from build123d import *

# Parameters (mm, degrees)
SKETCH1_W            = 12
SKETCH1_H            = 30
BOSS_EXTRUDE1_DEPTH  = 3
BOSS_EXTRUDE2_DEPTH  = 13
M5_CLEARANCE_HOLE1_D = 5.5
M4_CLEARANCE_HOLE1_D = 4.5


with BuildPart() as part:
    # Sketch1 → Boss-Extrude1 (new body)
    with BuildSketch(Plane.XY):
        with Locations((6, 15)):
            Rectangle(SKETCH1_W, SKETCH1_H)
        Polygon((12, 0), (0, 0), (0, -3), (30, -3), (30, 0), align=None)
    extrude(amount=BOSS_EXTRUDE1_DEPTH)

    # Sketch1_3 → Boss-Extrude2 (add)
    with BuildSketch(Plane.XY):
        Polygon((12, 0), (0, 0), (0, -3), (30, -3), (30, 0), align=None)
    extrude(amount=-BOSS_EXTRUDE2_DEPTH)

    # Mirror1: part across plane


with BuildPart() as part_1:
    add(part.part)
    add(part.part.mirror(Plane.XY.offset(-13)))

    # M5 Clearance Hole1 (through all)
    with Locations(Plane(origin=(0, 0, 0), x_dir=(1, 0, 0), z_dir=(0, 1, 0))):
        with Locations((20, 13)):
            Hole(M5_CLEARANCE_HOLE1_D / 2)

    # M4 Clearance Hole1 (through all)
    with Locations(Plane.XY.offset(3)):
        with Locations((6, 24)):
            Hole(M4_CLEARANCE_HOLE1_D / 2)


solid = part_1.part
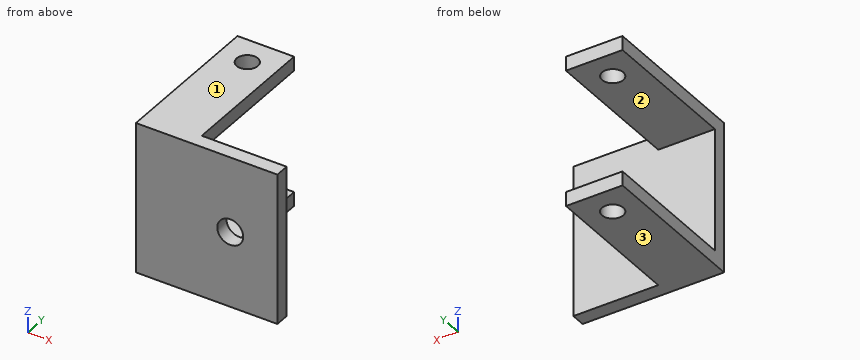
Geometry check sheet. Reference: the model listing, model coordinates, mm. Face numbers are marked on the shaded views. Round coordinates to 2 decimals unless told otherwise and drop trailing zeros. Loops run counter-clockwise (first coordinate to the right, second up) from the corner with the lowest first, then second, coordinate; pieces in that order, holes last.
Item 1: Cross-section at C-C on y = 24. Record the boundary of the cut face in (x, z).
Item 2: Gauge pin test, flat ends, axial feed: pin 1 (0.9 mm diameter, centred on y = 21, z = -27.5, fed in from +X); pin 2 (3.5 mm diameter, centred on x = 5.5, y = 22.5, fed in from -Z); pin 3 (6 mm diameter, centred on x = 23.5, z = -18, fed in from +Y). Record the tip position at first contact, or that the pin passes through.
Item 3: Thickness scan on line 1 (Z direction, x = 20, y = -1.6); line 2 (X direction, y = -1.5, z = -13); line 3 (Z direction, x = 3.5, y = 27.5). Record the ranges inside material, lowest first.
Item 4: Cross-section at D-D on x = 6. Record the boundary of the cut face in (y, z), then the cut area to 3 significant figures.
Item 5: Cross-section at A-A on x = 20. Record the boundary of the cut face in (y, z).
Item 6: Cross-section at B-B on y = 1.5. Record the boundary of the cut face in (x, z), then the cut area to 3 significant figures.
Item 7: Mould release check, pull along Z, two halves, no side actions. Record for the marked faces 1, 2 and 3: pulls with the +Z half, pulls with the -Z half, needs draft (parallel to the pull), parting line crosses it, or undercut.
Answer sheet:
1. outline: (0, -29) - (3.75, -29) - (3.75, -26) - (0, -26) - close; (0, 0) - (3.75, 0) - (3.75, 3) - (0, 3) - close; (8.25, -29) - (12, -29) - (12, -26) - (8.25, -26) - close; (8.25, 0) - (12, 0) - (12, 3) - (8.25, 3) - close
2. pin 1: stops at x = 12
2. pin 2: stops at z = -29
2. pin 3: stops at y = 0
3. line 1: z = -29 to -15.75, -10.25 to 3
3. line 2: x = 0 to 17.25, 22.75 to 30
3. line 3: z = -29 to -26, 0 to 3
4. outline: (-3, -29) - (21.75, -29) - (21.75, -26) - (0, -26) - (0, 0) - (21.75, 0) - (21.75, 3) - (-3, 3) - close; (26.25, -29) - (30, -29) - (30, -26) - (26.25, -26) - close; (26.25, 0) - (30, 0) - (30, 3) - (26.25, 3) - close
4. area: 249 mm2
5. outline: (-3, -29) - (0, -29) - (0, -15.75) - (-3, -15.75) - close; (-3, -10.25) - (0, -10.25) - (0, 3) - (-3, 3) - close
6. outline: (0, -29) - (12, -29) - (12, -26) - (0, -26) - close; (0, 0) - (12, 0) - (12, 3) - (0, 3) - close
6. area: 72.0 mm2
7. face 1: pulls with the +Z half
7. face 2: undercut
7. face 3: pulls with the -Z half
